from build123d import *

# Parameters (mm, degrees)
SKETCH1_W           = 35
SKETCH1_H           = 40
BOSS_EXTRUDE1_DEPTH = 10
FILLET1_R           = 3
SKETCH2_W           = 24
SKETCH2_H           = 2
BOSS_EXTRUDE2_DEPTH = 34
FILLET2_R           = 1
FILLET3_R           = 1


with BuildPart() as part:
    # Sketch1 → Boss-Extrude1 (new body)
    with BuildSketch(Plane.XY):
        with Locations((17.5, 20)):
            Rectangle(SKETCH1_W, SKETCH1_H)
    extrude(amount=BOSS_EXTRUDE1_DEPTH)

    # Fillet1
    fillet1_edges = [part.edges().sort_by_distance(p)[0] for p in [
        (0, 40, 5),
        (35, 40, 5),
    ]]
    fillet(fillet1_edges, radius=FILLET1_R)

    # Sketch2 → Boss-Extrude2 (add)
    with BuildSketch(Plane.XZ):
        with Locations((17.5, -1)):
            Rectangle(SKETCH2_W, SKETCH2_H)
    extrude(amount=-BOSS_EXTRUDE2_DEPTH)

    # Fillet2
    fillet2_edges = [part.edges().sort_by_distance(p)[0] for p in [
        (5.5, 34, -1),
        (5.5, 17, -2),
        (17.5, 34, 0),
        (5.5, 17, 0),
        (29.5, 34, -1),
        (29.5, 17, 0),
        (17.5, 34, -2),
        (29.5, 17, -2),
    ]]
    fillet(fillet2_edges, radius=FILLET2_R - 0.0001)  # a hair under: the kernel refuses the full size

    # Fillet3
    fillet3_edges = [part.edges().sort_by_distance(p)[0] for p in [
        (35, 18.5, 10),
        (0, 18.5, 0),
        (0, 18.5, 10),
        (17.5, 40, 0),
        (34.121320344, 39.121320344, 0),
        (0.878679656, 39.121320344, 0),
        (17.5, 40, 10),
        (34.121320344, 39.121320344, 10),
        (0.878679656, 39.121320344, 10),
        (32.74995, 0, 0),
        (17.5, 0, -2),
        (29.207136071, 0, -1.707136071),
        (5.792863929, 0, -1.707136071),
        (5.207136071, 0, -0.292863929),
        (29.792863929, 0, -0.292863929),
        (35, 18.5, 0),
        (2.25005, 0, 0),
        (17.5, 0, 10),
        (35, 0, 5),
        (0, 0, 5),
    ]]
    fillet(fillet3_edges, radius=FILLET3_R - 0.0001)  # a hair under: the kernel refuses the full size


solid = part.part
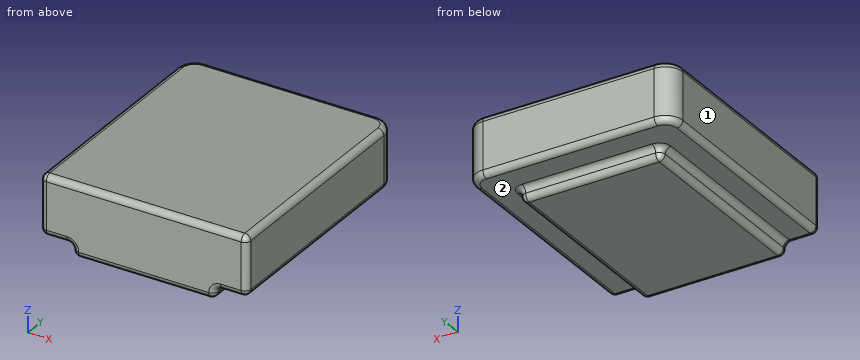
The listing builds one solid part. Answer for the finished solid, in the listing's coordinates (mm). Face numbers are marked on the shaded views. A direction names the side the tool comes from. Give positions to 0.01 mm unless a question says otherwise; leave off trailing zeros. Write each loop counter-clockwise with the first axis right and the second up, starting at its lowest first coordinate (ties: lowest second). Pieces come first, ordered by that corner, then holes.
Item 1: Which of the six approach directions +Z, -Z, +X, -X, +Y, -Y give full straight-line access (tool end or side, diameter ignored) to the marked faces 1 and 2?
Item 2: Find the intervals of material crossed by line 1 along Z through (x, y) = (10, 36.5); line 2 along Y through (x, z) = (23, -1.25); line 3 along Y through (x, z) = (33, 2), in increasing order.
Item 3: Section B-B, the plane x = 3.5 is taken. Write down the section's boundary in (y, z).
Completed:
1. face 1: +Z, -Z, -X, +Y, -Y
1. face 2: -Z, +Y
2. line 1: z = 0 to 10
2. line 2: y = 0.03 to 33.97
2. line 3: y = 0 to 39.83
3. outline: (0, 1) arc R1 ccw to (1, 0) - (39, 0) arc R1 ccw to (40, 1) - (40, 9) arc R1 ccw to (39, 10) - (1, 10) arc R1 ccw to (0, 9) - close
